Part model, mm, in its own coordinate system. Face numbers are marked on the shaded views. A direction names the side the tool comes from. Give positions to 0.01 mm unless a question says otherwise; leave off trailing zeros. Write each loop counter-clockwise with the first axis right and the second up, starting at its lowest first coordinate (ties: lowest second). Pieces come first, ordered by that corner, then holes. Notation, with made-up numbers: (41, 89) - (77, 89) arc R12 ccw to (77, 106) - close; hole circle Ø10 at (28, 49.5). An arc over 180 degrees is marked (long way). Answer in a Markdown table with one row per item. Add a question column.
1. Drop flat-ended pins along their axis: pin 1 Ø1.2 at (x, y) = (-43.5, 4.5) entering from +Z; pin 2 Ø7 at (x, z) = (-9, -60) entering from +Y; pin 3 Ø2 at (x, y) = (10.5, 4) entering from -Z; pin 4 Ø4 at (x, z) = (-16, 48.5) entering from -Y. Give the stop position or say it passes through.
2. Band-saw the part on D-D on x = -112.5. Write the cut outline in (y, z).
3. Probe line 1 along Z through (x, y) = (50, 1.3); line 2 along X through (y, z) = (0.35, -23.5); line 3 along X through (y, z) = (1, -31.5). List the from-to ranges inside material, lowest first.
4. Band-saw the part on B-B on x = 8. Write the cut outline in (y, z).
5. Band-saw the part on A-A on y = 1.35. Write the cut outline in (x, z), plus the area to 3 significant figures.
6. Which spindle directions (+Z, -Z, +X, -X, +Y, -Y) get a long thin tool onto all of the face, cutting with end or side? Do the marked faces 1 and 2. Say none if no direction does.
7. Pull direction Z, two halves, no side cores. Call the marked faces 3 and 4: released by +Z, released by -Z, zero draft, split by the parting line, or undercut.
8. Band-saw the part on C-C on z = -28. Write the cut outline in (x, y).
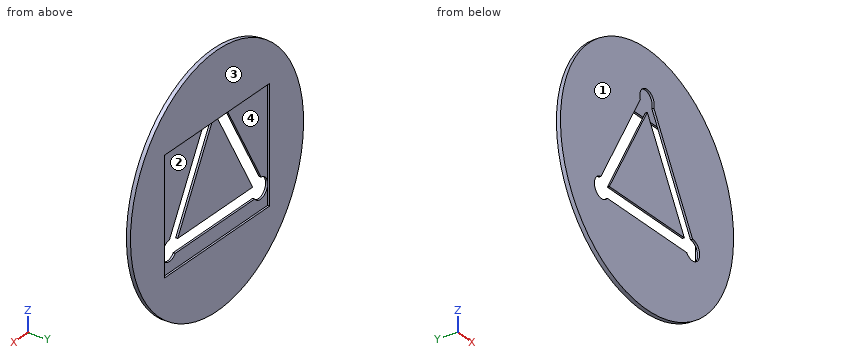
```python
from build123d import *

# Parameters (mm, degrees)
SKETCH1_R           = 150
BOSS_EXTRUDE1_DEPTH = 5
SKETCH2_R           = 12.5
CUT_EXTRUDE1_DEPTH  = 2.5
SKETCH4_W           = 182
SKETCH4_H           = 141
CUT_EXTRUDE2_DEPTH  = 2.5
CUT_EXTRUDE3_DEPTH  = 2.5


with BuildPart() as part:
    # Sketch1 → Boss-Extrude1 (new body)
    with BuildSketch(Plane(origin=(0, 0, 0), x_dir=(1, 0, 0), z_dir=(0, 1, 0))):
        with Locations(Location((0, 0, 0), (0, 0, 270))):
            Circle(SKETCH1_R)
    extrude(amount=BOSS_EXTRUDE1_DEPTH)

    # Sketch2 → Cut-Extrude1 (cut)
    with BuildSketch(Plane.XZ):
        with Locations(Location((0, 90.907224223, 0), (0, 0, 270))):
            Circle(SKETCH2_R)
        with Locations(Location((78.727965565, -45.453612112, 0), (0, 0, 270))):
            Circle(SKETCH2_R)
        with Locations(Location((-78.727965565, -45.453612112, 0), (0, 0, 270))):
            Circle(SKETCH2_R)
    extrude(amount=-CUT_EXTRUDE1_DEPTH, mode=Mode.SUBTRACT)

    # Sketch4 → Cut-Extrude2 (cut)
    with BuildSketch(Plane(origin=(0, 5, 0), x_dir=(1, 0, 0), z_dir=(0, 1, 0))):
        Rectangle(SKETCH4_W, SKETCH4_H)
    extrude(amount=-CUT_EXTRUDE2_DEPTH, mode=Mode.SUBTRACT)

    # Sketch5 → Cut-Extrude3 (cut)
    with BuildSketch(Plane.XZ):
        with BuildLine():
            Line((-11.659324393, 86.400545325), (-79.955582896, -33.014039945))
            ThreePointArc((-79.955582896, -33.014039945), (-67.813794545, -39.360101552), (-68.782668785, -53.0260009))
            Line((-68.782668785, -53.0260009), (68.782668785, -53.0260009))
            ThreePointArc((68.782668785, -53.0260009), (67.573694856, -39.811604938), (78.934736548, -32.955322398))
            Line((78.934736548, -32.955322398), (11.934955449, 87.191468792))
            ThreePointArc((11.934955449, 87.191468792), (0.418787658, 78.414241517), (-11.659324393, 86.400545325))
        make_face()
        Polygon((0.484780027, 77.168816505), (-65.315283199, -37.881223324), (64.642360996, -37.881223324), align=None, mode=Mode.SUBTRACT)
    extrude(amount=-CUT_EXTRUDE3_DEPTH, mode=Mode.SUBTRACT)


solid = part.part
```
Values:
| question | item | result |
|---|---|---|
| 1 | pin 1 | stops at z = 143.73 |
| 1 | pin 2 | stops at y = 2.5 |
| 1 | pin 3 | stops at z = -149.7 |
| 1 | pin 4 | stops at y = 0 |
| 2 | outline | (0, -99.22) - (5, -99.22) - (5, 99.22) - (0, 99.22) - close |
| 3 | line 1 | z = -141.42 to -53.03, -37.88 to -11.62, 18.93 to 141.42 |
| 3 | line 2 | x = -148.15 to -74.51, -57.09 to 56.62, 73.66 to 148.15 |
| 3 | line 3 | x = -146.66 to -79.09, -61.67 to 61.08, 78.12 to 146.66 |
| 4 | outline | (0, -149.79) - (5, -149.79) - (5, -70.5) - (2.5, -70.5) - (2.5, -53.03) - (0, -53.03) - close; (0, -37.88) - (2.5, -37.88) - (2.5, 63.69) - (0, 63.69) - close; (0, 100.51) - (2.5, 100.51) - (2.5, 70.5) - (5, 70.5) - (5, 149.79) - (0, 149.79) - close |
| 5 | outline | circle Ø300 at (0, 0); (-65.32, -37.88) - (64.64, -37.88) - (0.48, 77.17) - close; hole (-79.96, -33.01) arc R12.5 ccw (long way) to (-68.78, -53.03) - (68.78, -53.03) arc R12.5 ccw (long way) to (78.93, -32.96) - (11.93, 87.19) arc R12.5 ccw (long way) to (-11.66, 86.4) - close |
| 5 | area | 63,200 mm² |
| 6 | face 1 | +Z, -Z, +X, -X, -Y |
| 6 | face 2 | +Y |
| 7 | face 3 | zero draft |
| 7 | face 4 | undercut |
| 8 | outline | (-147.36, 0) - (-77.09, 0) - (-77.09, 2.5) - (-91, 2.5) - (-91, 5) - (-147.36, 5) - close; (-59.66, 0) - (59.13, 0) - (59.13, 2.5) - (-59.66, 2.5) - close; (76.17, 0) - (147.36, 0) - (147.36, 5) - (91, 5) - (91, 2.5) - (76.17, 2.5) - close |
